Here's how the part is built. I have some questions about the finished solid (model axes, mm). A direction names the side the tool comes from. Coordinates: 2 decimals unless noted, no trailing zeros. Write each loop counter-clockwise with the first axis right and the second up, starting at its lowest first coordinate (ties: lowest second). Pieces come first, ordered by that corner, then holes. Notation, with made-up numbers: (19.5, -16) - (28.5, -16) arc R20 cw to (28.5, 16) - close; hole circle Ø5 at (6.25, 4.5). An arc over 180 degrees is marked (long way). Answer in a Markdown table with one row per item. Add a question column.
Item 1: Imagine slicing it at C-C (x = -5). Please give me the cut outline in (y, z).
Item 2: If I drill on probe 1 along Y at (x, z) = (105, 1) (3 decimals); probe 2 along Y at (x, z) = (70, 5.5); probe 3 along X at (y, z) = (3.5, 2.75), over which ranges is the centre line in solid material (lowest first)? Write a range as from..to.
Item 3: Which directions (+Z, -Z, +X, -X, +Y, -Y) give clear straight access to the entire face, cutting with the end or side of a thin tool? Please do faces 4 (the face through (51, 0, 0)), 5 (the face through (100, 0, 4)).
Item 4: Imagine slicing it at A-A (y = 0). Please give me the cut outline in (x, z), plus the area to 3 significant figures.
Item 5: I'm going to push flat-ended pins straight in: pin 1 (3 mm diameter, centred on y = 15, z = 6, fed in from -X); pin 2 (11.5 mm diameter, centred on x = 0, y = 0, fed in from -Z); pin 3 (1.9 mm diameter, centred on y = 0, z = 4.5, fed in from +X); pin 4 (1 mm diameter, centred on y = -6, z = 3.5, fed in from -X). Where does each tip first touch, or does it pass through?
Item 6: Imagine slicing it at B-B (z = 4). Please give me the cut outline in (x, y) (3 decimals), plus the area to 3 significant figures.
Item 7: We'd pull the mould along X, two halves only. Please class faces 1 (the face through (76.057, 1.907, 3.913)), 2 (the face through (-19.045, -0.419, 3.913)), 3 (the face through (110, -3.175, 4)): +X half, -X half, draft (parallel to the pull), parting line (faces both ways), or undercut.
from build123d import *

# Parameters (mm, degrees)
SKETCH1_R           = 6.35
BOSS_EXTRUDE1_DEPTH = 7.9375


with BuildPart() as part:
    # Sketch1 → Boss-Extrude1 (new body)
    with BuildSketch(Plane.XY):
        with BuildLine():
            Line((0, 19.05), (120, 19.05))
            Line((120, 19.05), (120, 3.175))
            Line((120, 3.175), (100, 3.175))
            Line((100, 3.175), (100, -3.175))
            Line((100, -3.175), (120, -3.175))
            Line((120, -3.175), (120, -19.05))
            Line((120, -19.05), (0, -19.05))
            ThreePointArc((0, -19.05), (-19.05, 0), (0, 19.05))
        make_face()
        Circle(SKETCH1_R, mode=Mode.SUBTRACT)
        with Locations((70, 0)):
            Circle(SKETCH1_R, mode=Mode.SUBTRACT)
    extrude(amount=BOSS_EXTRUDE1_DEPTH)


solid = part.part
Here are the results:
| question | item | result |
|---|---|---|
| 1 | outline | (-18.38, 0) - (-3.91, 0) - (-3.91, 7.94) - (-18.38, 7.94) - close; (3.91, 0) - (18.38, 0) - (18.38, 7.94) - (3.91, 7.94) - close |
| 2 | probe 1 | y = -19.05..-3.175, 3.175..19.05 |
| 2 | probe 2 | y = -19.05..-6.35, 6.35..19.05 |
| 2 | probe 3 | x = -18.73..-5.3, 5.3..64.7, 75.3..120 |
| 3 | face 4 | -Z, +X, -X, +Y, -Y |
| 3 | face 5 | +Z, -Z, +X |
| 4 | outline | (-19.05, 0) - (-6.35, 0) - (-6.35, 7.94) - (-19.05, 7.94) - close; (6.35, 0) - (63.65, 0) - (63.65, 7.94) - (6.35, 7.94) - close; (76.35, 0) - (100, 0) - (100, 7.94) - (76.35, 7.94) - close |
| 4 | area | 743 mm2 |
| 5 | pin 1 | stops at x = -13.44 |
| 5 | pin 2 | passes through |
| 5 | pin 3 | stops at x = 100 |
| 5 | pin 4 | stops at x = -18.24 |
| 6 | outline | (0, -19.05) - (120, -19.05) - (120, -3.175) - (100, -3.175) - (100, 3.175) - (120, 3.175) - (120, 19.05) - (0, 19.05) arc R19.05 ccw to start; hole circle Ø12.7 at (0, 0); hole circle Ø12.7 at (70, 0) |
| 6 | area | 4,760 mm2 |
| 7 | face 1 | undercut |
| 7 | face 2 | -X half |
| 7 | face 3 | draft |
